The listing builds one solid part. Answer for the finished solid, in the listing's coordinates (mm). Round coordinates to 2 decimals unless told otherwise and drop trailing zeros. Write each loop counter-clockwise with the first axis right and the second up, starting at its lowest first coordinate (ties: lowest second). Pieces come first, ordered by that corner, then holes. Notation, with made-up numbers: (45.5, -37.5) - (52.5, -37.5) arc R23 cw to (52.5, -21.5) - close; hole circle Ø4 at (-24, -37). An arc over 180 degrees is marked (long way). Use a Markdown table: item, result. Add a question column.
1) A cutting plane is placed at A-A (z = -3.75). Give the vertices of the cut face in (x, y), then the cut area to 3 significant figures.
2) This flat-tipped pin is pushed along its axis until it touches: P1, Ø1.5, axis at y = -1.5, z = -1.5, coming from the +X side. Where does it stop, or does it pass through?
3) Find the intervals of material crossed by probe 1 along Z at (x, y) = (0.9, -3.75); probe 2 along Y at (x, z) = (5.75, 1.1); probe 3 along X at (y, z) = (-0.25, -5.75), in increasing order. Write a range as from..to.
4) Determine the mould class of faces 1 (the cylindrical face through (5.37, -2.04, 0.99)), 2 (the flat face through (7, -2, 0)), 3 (the flat face through (2, -5.5, -4.5)) for opening direction X: +X half, -X half, draft (parallel to the pull), parting line (faces both ways), or undercut.
5) A cutting plane is placed at B-B (x = 5.75). Give the vertices of the cut face in (y, z), then the cut area to 3 significant figures.
6) A cutting plane is placed at D-D (x = 0.5). Give the vertices of the cut face in (y, z), then the cut area to 3 significant figures.
7) A cutting plane is placed at C-C (y = -3.75). Give the vertices of the cut face in (x, z), then the cut area to 3 significant figures.
Autodesk Inventor part; units mm, degrees
ref_plane "YZ Plane" through (0, 0, 0) normal (1, 0, 0) x (0, 1, 0)
ref_plane "XZ Plane" through (0, 0, 0) normal (0, 1, 0) x (-1, 0, 0)
ref_plane "XY Plane" through (0, 0, 0) normal (0, 0, 1) x (1, 0, 0)
sketch "Boceto1" plane through (0, 0, 0) normal (1, 0, 0) x (0, 1, 0)
  line L0 (0, 0) -> (0, -2)
  line L1 (0, -2) -> (0, -5.5)
  line L2 (0, -5.5) -> (0, -7.5)
  line L3 (0, -7.5) -> (-2, -7.5)
  line L4 (-2, -7.5) -> (-5.5, -7.5)
  line L5 (0, 0) -> (-5.5, 0)
  line L6 (-5.5, -7.5) -> (-7.5, -7.5)
  line L7 (-7.5, -7.5) -> (-7.5, 0)
  line L8 (-7.5, 0) -> (0, 0)
  circle A0 centre (-3.75, -3.75) radius 1.75
  dimension "d0" = 2
  dimension "d1" = 3.5
  dimension "d2" = 2
  dimension "d3" = 2
  dimension "d4" = 3.5
  dimension "d5" = 2
sketch "Boceto2" plane through (0, 0, 0) normal (0, 0, 1) x (1, 0, 0)
  line L0 (0, 0) -> (2, 0)
  line L1 (2, 0) -> (2, -7.5)
  line L2 (2, 0) -> (3, 0)
  line L3 (2.8119, -7.5) -> (0, -7.5)
  line L4 (0, -7.5) -> (0, 0)
  line L5 (3, 0) -> (3, -7.5)
  line L6 (3, -7.5) -> (0, -7.5)
  line L7 (3, 0) -> (6.5, 0)
  line L8 (6.5, 0) -> (8.5, 0)
  line L9 (8.5, 0) -> (8.5, -7.5)
  line L10 (8.5, -7.5) -> (3, -7.5)
  circle A0 centre (5.75, -3.75) radius 1.75
  dimension "d6" = 2
  dimension "d15" = 1
  dimension "d16" = 3.5
  dimension "d17" = 2
  dimension "d18" = 3.5
extrude "Extrusión1" add sketch "Boceto1" along normal blind 2
extrude "Extrusión2" add sketch "Boceto2" along normal blind 2
sketch "Boceto4" plane through (0, 0, 2) normal (0, 0, 1) x (1, 0, 0)
  line L0 (8.5, -7.5) -> (9.5, -7.5)
  line L1 (9.5, -7.5) -> (9.5, 0)
  line L2 (9.5, 0) -> (8.5, 0)
  line L3 (8.5, -7.5) -> (8.5, 0)
  line L4 (8.5, 0) -> (8.5, -7.5)
  point P0 (0, 0)
  dimension "d24" = 1
extrude "Extrusión3" add sketch "Boceto4" against normal blind 2
properties part number "Pantalla - tirado 90gr"
Entries:
| question | item | result |
|---|---|---|
| 1 | outline | (0, -7.5) - (2, -7.5) - (2, -5.5) - (0, -5.5) - close; (0, -2) - (2, -2) - (2, 0) - (0, 0) - close |
| 1 | area | 8.00 mm² |
| 2 | P1 | stops at x = 2 |
| 3 | probe 1 | z = -7.5..-5.5, -2..2 |
| 3 | probe 2 | y = -7.5..-5.5, -2..0 |
| 3 | probe 3 | x = 0..2 |
| 4 | face 1 | undercut |
| 4 | face 2 | draft |
| 4 | face 3 | +X half |
| 5 | outline | (-7.5, 0) - (-5.5, 0) - (-5.5, 2) - (-7.5, 2) - close; (-2, 0) - (0, 0) - (0, 2) - (-2, 2) - close |
| 5 | area | 8.00 mm² |
| 6 | outline | (-7.5, -7.5) - (0, -7.5) - (0, 2) - (-7.5, 2) - close; hole circle Ø3.5 at (-3.75, -3.75) |
| 6 | area | 61.6 mm² |
| 7 | outline | (0, -7.5) - (2, -7.5) - (2, -5.5) - (0, -5.5) - close; (0, -2) - (2, -2) - (2, 0) - (4, 0) - (4, 2) - (0, 2) - close; (7.5, 0) - (9.5, 0) - (9.5, 2) - (7.5, 2) - close |
| 7 | area | 20.0 mm² |
